Here's how the part is built. I have some questions about the finished solid (model axes, mm). Face numbers are marked on the shaded views. A direction names the side the tool comes from. Coordinates: 2 decimals unless noted, no trailing zeros. Write each loop counter-clockwise with the first axis right and the second up, starting at its lowest first coordinate (ties: lowest second). Pieces come first, ordered by that corner, then holes. Notation, with made-up numbers: (31.25, -19.5) -> (64.25, -19.5) arc R21 cw to (64.25, 11.5) -> close; hole circle Ø9 at (26, 67). An arc over 180 degrees is marked (long way). Put each result on its own line as item: value. Start each with the question number.
Item 1: I want a section at B-B, the plane y = -1.75. List the corners of the cut face in (x, z) for me.
Item 2: I want a section at D-D, the plane z = 5.75. List the corners of the cut face in (x, y) for me.
Item 3: If we mould it in two halves opening along Y, with no side actions, what happens to the marked faces 1, 2, 3 and 4? For each: released by +Y, released by -Y, zero draft, split by the parting line, or undercut.
Item 4: I want a section at C-C, the plane x = -4. List the corners of the cut face in (y, z) for me.
Item 5: I need wall thicknesses on line 1 (X direction, y = 2.5, z = 2); line 2 (Y direction, x = -10, z = 2); line 3 (Y direction, x = -2, z = 3.75). Which ranges of each line are inside material? Lowest first, please. Write a range as [from, to].
Item 6: For pin 1 (1.9 mm diameter, centred on x = 10.5, z = 4.5, fed in from +Y), with a flat end and sliding along its axis, tell me the tip position at first contact or that it passes through.
Item 7: I want a section at A-A, the plane z = 3. List the corners of the cut face in (x, y) for me.
Item 8: On a 3-axis mill with a long thin cutter (end or side, diameter ignored), from which of +Z, -Z, +X, -X, +Y, -Y can I reach the whole of each face in a straight line? I mean the marked faces 5 and 6. Say none if no direction works.
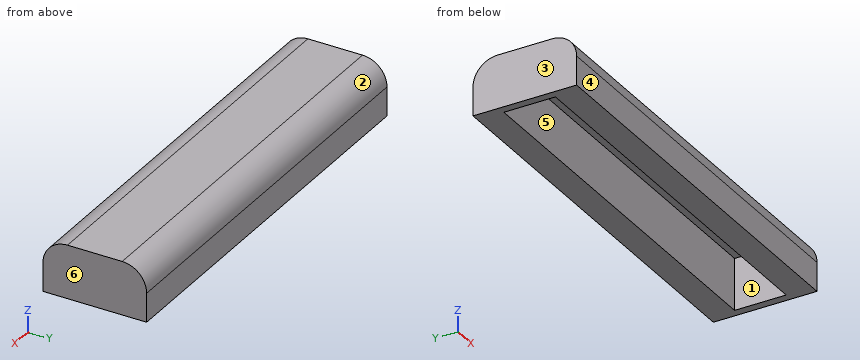
from build123d import *

# Parameters (mm, degrees)
SKETCH1_W           = 50
SKETCH1_H           = 12.7
BOSS_EXTRUDE1_DEPTH = 6.55
SKETCH2_W           = 48
SKETCH2_H           = 6.32
CUT_EXTRUDE2_DEPTH  = 6.35
FILLET1_R           = 3


with BuildPart() as part:
    # Sketch1 → Boss-Extrude1 (new body)
    with BuildSketch(Plane.XY):
        Rectangle(SKETCH1_W, SKETCH1_H)
    extrude(amount=BOSS_EXTRUDE1_DEPTH)

    # Sketch2 → Cut-Extrude2 (cut)
    with BuildSketch(Plane(origin=(0, 0, 0), x_dir=(-1, 0, 0), z_dir=(0, 0, -1))):
        Rectangle(SKETCH2_W, SKETCH2_H)
    extrude(amount=-CUT_EXTRUDE2_DEPTH, mode=Mode.SUBTRACT)

    # Fillet1
    fillet1_edges = [part.edges().sort_by_distance(p)[0] for p in [
        (0, 6.35, 6.55),
        (0, -6.35, 6.55),
    ]]
    fillet(fillet1_edges, radius=FILLET1_R)


solid = part.part
Calculated:
1. outline: (-25, 0) -> (-24, 0) -> (-24, 6.35) -> (24, 6.35) -> (24, 0) -> (25, 0) -> (25, 6.55) -> (-25, 6.55) -> close
2. outline: (-25, -5.39) -> (25, -5.39) -> (25, 5.39) -> (-25, 5.39) -> close; hole (-24, -3.16) -> (24, -3.16) -> (24, 3.16) -> (-24, 3.16) -> close
3. face 1: undercut
3. face 2: released by +Y
3. face 3: zero draft
3. face 4: released by -Y
4. outline: (-6.35, 0) -> (-3.16, 0) -> (-3.16, 6.35) -> (3.16, 6.35) -> (3.16, 0) -> (6.35, 0) -> (6.35, 3.55) arc R3 ccw to (3.35, 6.55) -> (-3.35, 6.55) arc R3 ccw to (-6.35, 3.55) -> close
5. line 1: x = [-25, -24], [24, 25]
5. line 2: y = [-6.35, -3.16], [3.16, 6.35]
5. line 3: y = [-6.34, -3.16], [3.16, 6.34]
6. pin 1: stops at y = 6.35
7. outline: (-25, -6.35) -> (25, -6.35) -> (25, 6.35) -> (-25, 6.35) -> close; hole (-24, -3.16) -> (24, -3.16) -> (24, 3.16) -> (-24, 3.16) -> close
8. face 5: -Z
8. face 6: +Z, -Z, +X, +Y, -Y
